Work out the finished part from the listing and answer in its coordinate system (mm). A direction names the side the tool comes from. Round coordinates to 2 decimals unless told otherwise and drop trailing zeros. Order: outer loops, then holes, each group sorted by start corner. A loop starts at its lowest first (then second) coordinate and runs counter-clockwise, first axis right, second up. Notation, with made-up numbers: (50, -7) -> (63, -7) arc R21 cw to (63, 18) -> close; hole circle Ø8 at (88.25, 69.5). An arc over 180 degrees is marked (long way). Use a Markdown table: item, result. Add a question column.
Item 1: For a pull along X with two mould halves and no side action, classify faces 1 (the cylindrical face through (28.753, 9.022, 4.159)), 2 (the cylindrical face through (-37, 29.4, 7.5)), 3 (the flat face through (-37.3, 17.98, 8.2)) as +X half, -X half, draft (parallel to the pull), parting line (faces both ways), or undercut.
Item 2: A cutting plane is placed at C-C, the plane x = 17.5. Determine the outline of the cut face in (y, z), plus the area to 3 significant figures.
Item 3: Flat-ended cylindrical pins translate along their axes: P1, Ø0.8, axis at x = -37, y = 12, coming from the +Z side; P2, Ø5, axis at x = -12.5, y = 8, coming from the +Z side; P3, Ø4, axis at x = 31.75, y = -19.05, coming from the +Z side. Find the tip coordinate at first contact, or state that the pin passes through.
Item 4: A cutting plane is placed at D-D, the plane y = -2. Determine the outline of the cut face in (x, z), plus the area to 3 significant figures.
Item 5: Find the intervals of material crossed by L1, parallel to Y at x = 31.75, z = 4.2; L2, parallel to Y at x = -19.05, z = 3.7; L3, parallel to Y at x = 33, z = 9, in increasing order. Write a range as [from, to].
Item 6: A cutting plane is placed at A-A, the plane z = 9. Determine the outline of the cut face in (x, y).
Item 7: A tool of negligible diameter and unlimited length cuts with its end or side. For faces 4 (the cylindrical face through (-17.46, -23.23, 4.15)), 5 (the cylindrical face through (0.488, -29.067, 1.141)), 6 (the flat face through (-37, -17, 6.49)), from which of +Z, -Z, +X, -X, +Y, -Y can it reach the whole face along a straight path? Write none if from no direction.
Item 8: A cutting plane is placed at B-B, the plane y = 24.13. Determine the outline of the cut face in (x, z).
from build123d import *

# Parameters (mm, degrees)
SKETCH001_W     = 75.78
SKETCH001_H     = 60.54
PAD_DEPTH       = 11
SKETCH002_W     = 72.58
SKETCH002_H     = 57.34
POCKET_DEPTH    = 9.8
SKETCH005_W     = 74.18
SKETCH005_H     = 58.94
POCKET001_DEPTH = 3
SKETCH003_R     = 3
SKETCH003_R_2   = 1.5
PAD001_DEPTH    = 4
SKETCH004_W     = 12.72
SKETCH004_H     = 10.8
SKETCH004_W_2   = 9.14
POCKET002_DEPTH = 5
FILLET_R        = 4
FILLET001_R     = 1
FILLET002_R     = 2
FILLET003_R     = 3
FILLET004_R     = 2


with BuildPart() as part:
    # Sketch001 → Pad (new body)
    with BuildSketch(Plane.XY):
        Rectangle(SKETCH001_W, SKETCH001_H)
    extrude(amount=PAD_DEPTH)

    # Sketch002 (on Face6 of Pad) → Pocket (cut)
    with BuildSketch(Plane.XY.offset(11)):
        Rectangle(SKETCH002_W, SKETCH002_H)
    extrude(amount=-POCKET_DEPTH, mode=Mode.SUBTRACT)

    # Sketch005 (on DatumPlane) → Pocket001 (cut)
    with BuildSketch(Plane.XY.offset(11)):
        Rectangle(SKETCH005_W, SKETCH005_H)
    extrude(amount=-POCKET001_DEPTH, mode=Mode.SUBTRACT)

    # Sketch003 (on Face11 of Pocket) → Pad001 (join)
    with BuildSketch(Plane.XY.offset(1.2)):
        with Locations((-19.05, 24.13)):
            Circle(SKETCH003_R)
        with Locations((-19.05, 24.13)):
            Circle(SKETCH003_R_2, mode=Mode.SUBTRACT)
        with Locations((31.75, 8.89)):
            Circle(SKETCH003_R)
        with Locations((31.75, 8.89)):
            Circle(SKETCH003_R_2, mode=Mode.SUBTRACT)
        with Locations((-20.32, -24.13)):
            Circle(SKETCH003_R)
        with Locations((-20.32, -24.13)):
            Circle(SKETCH003_R_2, mode=Mode.SUBTRACT)
        with Locations((31.75, -19.05)):
            Circle(SKETCH003_R)
        with Locations((31.75, -19.05)):
            Circle(SKETCH003_R_2, mode=Mode.SUBTRACT)
    extrude(amount=PAD001_DEPTH)

    # Sketch004 (on Face2 of Pad001) → Pocket002 (cut)
    with BuildSketch(Plane(origin=(-37.89, 0, 0), x_dir=(0, -1, 0), z_dir=(-1, 0, 0))):
        with Locations((-11.62, 11.89)):
            Rectangle(SKETCH004_W, SKETCH004_H)
        with Locations((16.69, 11.89)):
            Rectangle(SKETCH004_W_2, SKETCH004_H)
    extrude(amount=-POCKET002_DEPTH, mode=Mode.SUBTRACT)

    # Fillet
    fillet_edges = [part.edges().sort_by_distance(p)[0] for p in [
        (0, 30.27, 0),
        (37.89, 0, 0),
        (0, -30.27, 0),
        (-37.89, 0, 0),
    ]]
    fillet(fillet_edges, radius=FILLET_R)

    # Fillet001
    fillet001_edges = [part.edges().sort_by_distance(p)[0] for p in [
        (36.29, 28.67, 4.6),
        (36.29, -28.67, 4.6),
        (-36.29, -28.67, 4.6),
        (-36.29, 28.67, 4.6),
    ]]
    fillet(fillet001_edges, radius=FILLET001_R)

    # Fillet002
    fillet002_edges = [part.edges().sort_by_distance(p)[0] for p in [
        (-37.09, -29.47, 9.5),
        (-37.09, 29.47, 9.5),
        (37.09, 29.47, 9.5),
        (37.09, -29.47, 9.5),
    ]]
    fillet(fillet002_edges, radius=FILLET002_R)

    # Fillet003
    fillet003_edges = [part.edges().sort_by_distance(p)[0] for p in [
        (-37.89, -30.27, 7.5),
        (37.89, -30.27, 7.5),
        (37.89, 30.27, 7.5),
        (-37.89, 30.27, 7.5),
    ]]
    fillet(fillet003_edges, radius=FILLET003_R)

    # Fillet004
    fillet004_edges = [part.edges().sort_by_distance(p)[0] for p in [
        (-22.05, 24.13, 1.2),
        (28.75, 8.89, 1.2),
        (28.75, -19.05, 1.2),
        (-23.32, -24.13, 1.2),
    ]]
    fillet(fillet004_edges, radius=FILLET004_R)


solid = part.part
Reported:
| question | item | result |
|---|---|---|
| 1 | face 1 | undercut |
| 1 | face 2 | -X half |
| 1 | face 3 | draft |
| 2 | outline | (-30.27, 4) arc R4 ccw to (-26.27, 0) -> (26.27, 0) arc R4 ccw to (30.27, 4) -> (30.27, 11) -> (29.47, 11) -> (29.47, 8) -> (28.67, 8) -> (28.67, 1.2) -> (-28.67, 1.2) -> (-28.67, 8) -> (-29.47, 8) -> (-29.47, 11) -> (-30.27, 11) -> close |
| 2 | area | 92.3 mm² |
| 3 | P1 | z = 6.49 |
| 3 | P2 | z = 1.2 |
| 3 | P3 | z = 5.2 |
| 4 | outline | (-37.89, 4) arc R4 ccw to (-33.89, 0) -> (33.89, 0) arc R4 ccw to (37.89, 4) -> (37.89, 11) -> (37.09, 11) -> (37.09, 8) -> (36.29, 8) -> (36.29, 1.2) -> (-36.29, 1.2) -> (-36.29, 8) -> (-37.09, 8) -> (-37.09, 11) -> (-37.89, 11) -> close |
| 4 | area | 111 mm² |
| 5 | L1 | [-30.27, -28.67], [-22.05, -20.55], [-17.55, -16.05], [5.89, 7.39], [10.39, 11.89], [28.67, 30.27] |
| 5 | L2 | [-30.26, -28.67], [-26.85, -24.93], [-23.33, -21.41], [21.13, 22.63], [25.63, 27.13], [28.67, 30.26] |
| 5 | L3 | [-30.27, -29.47], [29.47, 30.27] |
| 6 | outline | (-37.89, -27.27) arc R3 ccw to (-34.89, -30.27) -> (34.89, -30.27) arc R3 ccw to (37.89, -27.27) -> (37.89, 27.27) arc R3 ccw to (34.89, 30.27) -> (-34.89, 30.27) arc R3 ccw to (-37.89, 27.27) -> (-37.89, 17.98) -> (-37.09, 17.98) -> (-37.09, 27.47) arc R2 cw to (-35.09, 29.47) -> (35.09, 29.47) arc R2 cw to (37.09, 27.47) -> (37.09, -27.47) arc R2 cw to (35.09, -29.47) -> (-35.09, -29.47) arc R2 cw to (-37.09, -27.47) -> (-37.09, -21.26) -> (-37.89, -21.26) -> close; (-37.89, -12.12) -> (-37.09, -12.12) -> (-37.09, 5.26) -> (-37.89, 5.26) -> close |
| 7 | face 4 | +Z |
| 7 | face 5 | -Z, +X, -X, -Y |
| 7 | face 6 | +Z, -X |
| 8 | outline | (-37.89, 4) arc R4 ccw to (-33.89, 0) -> (33.89, 0) arc R4 ccw to (37.89, 4) -> (37.89, 11) -> (37.09, 11) -> (37.09, 8) -> (36.29, 8) -> (36.29, 1.2) -> (-14.05, 1.2) arc R2 cw to (-16.05, 3.2) -> (-16.05, 5.2) -> (-17.55, 5.2) -> (-17.55, 1.2) -> (-20.55, 1.2) -> (-20.55, 5.2) -> (-22.05, 5.2) -> (-22.05, 3.2) arc R2 cw to (-24.05, 1.2) -> (-36.29, 1.2) -> (-36.29, 8) -> (-37.09, 8) -> (-37.09, 11) -> (-37.89, 11) -> close |
